The model under review builds one solid part; all positions refer to its coordinate system, in mm. A direction names the side the tool comes from. Give positions to 0.01 mm unless a question says otherwise; leave off trailing zeros. Write each loop counter-clockwise with the first axis right and the second up, starting at its lowest first coordinate (ties: lowest second). Pieces come first, ordered by that corner, then holes.
from build123d import *

# Parameters (mm, degrees)
F1_DEPTH = 25
F2_T     = -2.5


with BuildPart() as f1:
    # F0 (on Top) → F1 (new body)
    with BuildSketch(Plane.XY):
        with BuildLine():
            ThreePointArc((0, 5), (1.464466, 1.464466), (5, 0))
            Line((5, 0), (8.007363, 0))
            ThreePointArc((8.007363, 0), (11.542897, 1.464466), (13.007363, 5))
            Line((13.007363, 5), (13.007363, 13.368118))
            ThreePointArc((13.007363, 13.368118), (13.886043, 15.489438), (16.007363, 16.368118))
            Line((16.007363, 16.368118), (18.897251, 16.368118))
            ThreePointArc((18.897251, 16.368118), (21.018571, 15.489438), (21.897251, 13.368118))
            Line((21.897251, 13.368118), (21.897251, 5))
            ThreePointArc((21.897251, 5), (23.361717, 1.464466), (26.897251, 0))
            Line((26.897251, 0), (32.005447, 0))
            ThreePointArc((32.005447, 0), (35.540981, 1.464466), (37.005447, 5))
            Line((37.005447, 5), (37.005447, 26.097955))
            ThreePointArc((37.005447, 26.097955), (35.540981, 29.633489), (32.005447, 31.097955))
            Line((32.005447, 31.097955), (5, 31.097955))
            ThreePointArc((5, 31.097955), (1.464466, 29.633489), (0, 26.097955))
            Line((0, 26.097955), (0, 5))
        make_face()
    extrude(amount=F1_DEPTH)

    # F2
    f2_openings = [f1.faces().sort_by_distance(p)[0] for p in [
        (18.666559, 16.805031, 25),
    ]]
    offset(amount=F2_T, openings=f2_openings)


solid = f1.part
1) Consider section C-C, the plane y = 21.5. Give the boundary of the cut face in (x, z), then the cut area to 3 significant figures.
2) To check wall thickness, follow probe 1 along X at (y, z) = (8, 8.25); probe 2 along Y at (x, z) = (8, 13.5); probe 3 along X at (y, z) = (14, 4.75). State the ranges of each line that lie inside material, in increasing order.
3) Consider section A-A, the plane y = 10. Give the boundary of the cut face in (x, z), then the cut area to 3 significant figures.
4) The part is to be moulded in two halves that separate along Y. For faces 4 (the flat face through (24.397, 9, 14)), 5 (the flat face through (21.897, 9, 12)), 6 (the flat face through (17, 16.368, 12)), say which applies: +Y half, -Y half, draft (parallel to the pull), parting line (faces both ways), or undercut.
5) Tool access review of faces 1 (the flat face through (37.005, 15, 12)), 2 (the flat face through (34.505, 15, 14)), 3 (the cylindrical face through (13.863, 15.466, 12.325)): name each direction out of +Z, -Z, +X, -X, +Y, -Y from which nothing blocks a thin tool from reaching the whole face with its end or side.
6) Insertion check: pin 1 (2 mm diameter, centred on x = 12, z = 6.5, fed in from -Y); pin 2 (0.9 mm diameter, centred on x = 17.5, z = 7.5, fed in from -Y); pin 3 (7 mm diameter, centred on x = 21, z = 16, fed in from -Y). Each pin has a flat end and moves straight along its axis. Give the tip position at first contact, or say it passes through.
7) Consider section D-D, the plane x = 7. Give the boundary of the cut face in (y, z), then the cut area to 3 significant figures.
Answer block:
1. outline: (0, 0) - (37.01, 0) - (37.01, 25) - (34.51, 25) - (34.51, 2.5) - (2.5, 2.5) - (2.5, 25) - (0, 25) - close
1. area: 205 mm2
2. probe 1: x = 0 to 2.5, 10.51 to 13.01, 21.9 to 24.4, 34.51 to 37.01
2. probe 2: y = 0 to 2.5, 28.6 to 31.1
2. probe 3: x = 0 to 2.5, 10.54 to 13.07, 21.83 to 24.36, 34.51 to 37.01
3. outline: (0, 0) - (13.01, 0) - (13.01, 25) - (10.51, 25) - (10.51, 2.5) - (2.5, 2.5) - (2.5, 25) - (0, 25) - close; (21.9, 0) - (37.01, 0) - (37.01, 25) - (34.51, 25) - (34.51, 2.5) - (24.4, 2.5) - (24.4, 25) - (21.9, 25) - close
3. area: 295 mm2
4. face 4: undercut
4. face 5: draft
4. face 6: -Y half
5. face 1: +Z, -Z, +X, +Y, -Y
5. face 2: +Z
5. face 3: +Z, -Z, -Y
6. pin 1: stops at y = 0.99
6. pin 2: stops at y = 16.37
6. pin 3: stops at y = 0.61
7. outline: (0, 0) - (31.1, 0) - (31.1, 25) - (28.6, 25) - (28.6, 2.5) - (2.5, 2.5) - (2.5, 25) - (0, 25) - close
7. area: 190 mm2
